```python
from build123d import *

# Parameters (mm, degrees)
SKETCH_1_R      = 2
SKETCH_1_R_2    = 1.5
SKETCH_1_R_3    = 5
SKETCH_1_R_4    = 0.95
SKETCH_1_W      = 8.2
SKETCH_1_H      = 4.2
EXTRUDE_1_DEPTH = 4
FILLET_1_R      = 4
FILLET_2_R      = 1


with BuildPart() as part:
    # 草图1 → 凸台-拉伸1 (new body)
    with BuildSketch(Plane.XY):
        with BuildLine():
            Line((-38.15, 66.25), (-38.15, 62.25))
            Line((-38.15, 62.25), (-39.45, 62.25))
            Line((-39.45, 62.25), (-39.45, 59.65))
            Line((-39.45, 59.65), (-38.15, 59.65))
            Line((-38.15, 59.65), (-38.15, 57.05))
            Line((-38.15, 57.05), (-35.15, 57.05))
            Line((-35.15, 57.05), (-35.15, 59.65))
            Line((-35.15, 59.65), (-33.85, 59.65))
            Line((-33.85, 59.65), (-33.85, 62.25))
            Line((-33.85, 62.25), (-35.15, 62.25))
            Line((-35.15, 62.25), (-35.15, 66.25))
            Line((-35.15, 66.25), (-25.65, 66.25))
            Line((-25.65, 66.25), (-25.65, 70.25))
            Line((-25.65, 70.25), (-17.65, 70.25))
            Line((-17.65, 70.25), (-17.65, 66.25))
            Line((-17.65, 66.25), (-8.15, 66.25))
            Line((-8.15, 66.25), (-8.15, 62.25))
            Line((-8.15, 62.25), (-9.45, 62.25))
            Line((-9.45, 62.25), (-9.45, 59.65))
            Line((-9.45, 59.65), (-8.15, 59.65))
            Line((-8.15, 59.65), (-8.15, 57.05))
            Line((-8.15, 57.05), (-5.15, 57.05))
            Line((-5.15, 57.05), (-5.15, 59.65))
            Line((-5.15, 59.65), (-3.85, 59.65))
            Line((-3.85, 59.65), (-3.85, 62.25))
            Line((-3.85, 62.25), (-5.15, 62.25))
            Line((-5.15, 62.25), (-5.15, 66.25))
            Line((-5.15, 66.25), (4.35, 66.25))
            Line((4.35, 66.25), (4.35, 57.55))
            Line((4.35, 57.55), (53.51460577, -41.768082641))
            ThreePointArc((53.51460577, -41.768082641), (38.475737517, -73.658373169), (10.85, -51.75))
            Line((10.85, -51.75), (-95.15, 57.55))
            Line((-95.15, 57.55), (-95.15, 66.25))
            Line((-95.15, 66.25), (-85.65, 66.25))
            Line((-85.65, 66.25), (-85.65, 70.25))
            Line((-85.65, 70.25), (-77.65, 70.25))
            Line((-77.65, 70.25), (-77.65, 66.25))
            Line((-77.65, 66.25), (-68.15, 66.25))
            Line((-68.15, 66.25), (-68.15, 62.25))
            Line((-68.15, 62.25), (-69.45, 62.25))
            Line((-69.45, 62.25), (-69.45, 59.65))
            Line((-69.45, 59.65), (-68.15, 59.65))
            Line((-68.15, 59.65), (-68.15, 57.05))
            Line((-68.15, 57.05), (-65.15, 57.05))
            Line((-65.15, 57.05), (-65.15, 59.65))
            Line((-65.15, 59.65), (-63.85, 59.65))
            Line((-63.85, 59.65), (-63.85, 62.25))
            Line((-63.85, 62.25), (-65.15, 62.25))
            Line((-65.15, 62.25), (-65.15, 66.25))
            Line((-65.15, 66.25), (-55.65, 66.25))
            Line((-55.65, 66.25), (-55.65, 70.25))
            Line((-55.65, 70.25), (-47.65, 70.25))
            Line((-47.65, 70.25), (-47.65, 66.25))
            Line((-47.65, 66.25), (-38.15, 66.25))
        make_face()
        with Locations((-20.262745434, 32.422010331)):
            Circle(SKETCH_1_R, mode=Mode.SUBTRACT)
        with Locations((6.598407643, -9.75)):
            Circle(SKETCH_1_R_2, mode=Mode.SUBTRACT)
        with Locations((33.35, -51.75)):
            Circle(SKETCH_1_R_3, mode=Mode.SUBTRACT)
        with Locations((33.35, -45.75)):
            Circle(SKETCH_1_R_4, mode=Mode.SUBTRACT)
        with Locations((33.35, -57.75)):
            Circle(SKETCH_1_R_4, mode=Mode.SUBTRACT)
        with Locations((-8.401592357, -9.75)):
            Rectangle(SKETCH_1_W, SKETCH_1_H, mode=Mode.SUBTRACT)
        Polygon((-57.254487093, 52.05), (-41.177109745, 52.05), (-16.214099548, 4.334114018), align=None, mode=Mode.SUBTRACT)
        Polygon((12.65644769, 4.86329261), (-24.797659566, 52.05), (-8.394400914, 52.05), align=None, mode=Mode.SUBTRACT)
    extrude(amount=EXTRUDE_1_DEPTH)

    # 圆角1
    fillet_1_edges = [part.edges().sort_by_distance(p)[0] for p in [
        (-57.254487093, 52.05, 2),
        (-41.177109745, 52.05, 2),
        (-8.394400914, 52.05, 2),
        (-24.797659566, 52.05, 2),
    ]]
    fillet(fillet_1_edges, radius=FILLET_1_R)

    # 圆角2
    fillet_2_edges = [part.edges().sort_by_distance(p)[0] for p in [
        (-16.214099548, 4.334114018, 2),
        (12.65644769, 4.86329261, 2),
    ]]
    fillet(fillet_2_edges, radius=FILLET_2_R)


solid = part.part
```
Check sheet for the modelled part. Datum: model origin and axes. Units: mm. A direction names the side the tool comes from. Round coordinates to 2 decimals unless told otherwise and drop trailing zeros. Loops run counter-clockwise (first coordinate to the right, second up) from the corner with the lowest first, then second, coordinate; pieces in that order, holes last. Notation, with made-up numbers: (-23, -24) - (-12, -24) arc R20 ccw to (-12, -16) - close; hole circle Ø9 at (1.25, 35.5). An arc over 180 degrees is marked (long way). Write item = value, one per line. Start each with the question number.
Q1. Thickness scan on L1, parallel to Y at x = -48.5, z = 3.4; L2, parallel to X at y = 20, z = 2.7; L3, parallel to Y at x = 5, z = 2.25. Record the ranges inside material, lowest first.
Q2. Depth check by flat-ended pin: P1, Ø1.5, axis at y = 6, z = 3.5, coming from the -X side; P2, Ø0.8, axis at y = 60.5, z = 2, coming from the +X side; P3, Ø0.7, axis at x = -39, z = 2.5, coming from the -Y side. Enter the tip coordinate at first touch or a pass-through.
Q3. Section check B-B (y = -34.5). Record the boundary of the cut face in (x, z), plus the area to 3 significant figures.
Q4. Section check A-A (z = 3.3). Count the separate pieces of the cut face and the enclosed holes in it, plus the area to 3 significant figures.
Q5. Access from +Z, -Z, +X, -X, +Y, -Y to the whole of each face (thin tool, end or side, straight path). Record for faces 4 (the face through (-90, 66.25, 2)), 5 (the face through (-38.15, 64, 2)), 6 (the face through (-2, -1, 0)), 7 (the face through (-52.146, 49.776, 2.028)), 8 (the face through (-17.65, 68, 2)).
Q6. Release check for a two-part mould opening along X. For faces 1 (the face through (4.35, 62, 2)), 2 (the face through (0, 66.25, 2)), 3 (the face through (-20.145, 49.733, 2.028)) record: pulls with the +X half, pulls with the -X half, needs draft (parallel to the pull), parting line crosses it, or undercut.
Derived:
q1.L1 = 9.45 to 41.87, 52.05 to 70.25
q1.L2 = -58.73 to -29.69, -24.41 to 0.64, 5.9 to 22.94
q1.L3 = -45.72 to 14.51, 22.03 to 56.24
q2.P1 = -45.88
q2.P2 = 4.35
q2.P3 = -0.71
q3.outline = (-5.88, 0) - (49.92, 0) - (49.92, 4) - (-5.88, 4) - close
q3.area = 223 mm^2
q4.separate_pieces = 1
q4.enclosed_holes = 8
q4.area = 8,820 mm^2
q5.face_4 = +Z, -Z, -X, +Y
q5.face_5 = +Z, -Z, +Y
q5.face_6 = -Z, +X, -X, +Y, -Y
q5.face_7 = +Z, -Z
q5.face_8 = +Z, -Z, +X, +Y
q6.face_1 = pulls with the +X half
q6.face_2 = needs draft
q6.face_3 = undercut
